Work out the finished part from the listing and answer in its coordinate system (mm). Face numbers are marked on the shaded views. A direction names the side the tool comes from. Coordinates: 2 decimals unless noted, no trailing zeros. Order: outer loops, then holes, each group sorted by start corner. A loop starts at its lowest first (then second) coordinate and runs counter-clockwise, first axis right, second up. Notation, with made-up numbers: (-28.5, 5) -> (-22.5, 5) arc R16 cw to (-22.5, 28) -> close; hole circle Ø11 at (-2, -38.75). An arc over 180 degrees is marked (long way). Use one line per item in the form item = value.
from build123d import *

# Parameters (mm, degrees)
SKETCH1_W                                       = 60
SKETCH1_H                                       = 120
BOSS_EXTRUDE1_DEPTH                             = 6.54
SKETCH10_W                                      = 6.54
SKETCH10_H                                      = 45
BOSS_EXTRUDE5_DEPTH                             = 17
SKETCH17_W                                      = 60
SKETCH17_H                                      = 40
BOSS_EXTRUDE6_DEPTH                             = 29
CUT_EXTRUDE1_REACH                              = 42
CUT_EXTRUDE2_REACH                              = 54.54
SKETCH21_W                                      = 37.9445377
SKETCH21_H                                      = 40
SKETCH23_W                                      = 2
SKETCH23_H                                      = 36
CUT_EXTRUDE3_DEPTH                              = 9
SKETCH24_W                                      = 2
SKETCH24_H                                      = 36
CUT_EXTRUDE4_DEPTH                              = 9
CSK_FOR_M3_FLAT_HEAD_MACHINE_SCREW4_D           = 4.93
CSK_FOR_M3_FLAT_HEAD_MACHINE_SCREW4_DEPTH       = 6.54
CSK_FOR_M3_FLAT_HEAD_MACHINE_SCREW4_CSINK_D     = 12
CSK_FOR_M3_FLAT_HEAD_MACHINE_SCREW4_CSINK_ANGLE = 90
CSK_FOR_M3_FLAT_HEAD_MACHINE_SCREW5_D           = 4.93
CSK_FOR_M3_FLAT_HEAD_MACHINE_SCREW5_DEPTH       = 6.54
CSK_FOR_M3_FLAT_HEAD_MACHINE_SCREW5_CSINK_D     = 12
CSK_FOR_M3_FLAT_HEAD_MACHINE_SCREW5_CSINK_ANGLE = 90
BOSS_EXTRUDE8_DEPTH                             = 29
SKETCH36_W                                      = 60
SKETCH36_H                                      = 1.8
BOSS_EXTRUDE9_DEPTH                             = 6.5
FILLET1_R                                       = 3
FILLET2_R                                       = 2


with BuildPart() as part:
    # Sketch1 → Boss-Extrude1 (new body)
    with BuildSketch(Plane.XY):
        Rectangle(SKETCH1_W, SKETCH1_H)
    extrude(amount=BOSS_EXTRUDE1_DEPTH)

    # Sketch10 → Boss-Extrude5 (add)
    with BuildSketch(Plane(origin=(0, 0, 0), x_dir=(-1, 0, 0), z_dir=(0, 0, -1))):
        with Locations((23.27, -2.5)):
            Rectangle(SKETCH10_W, SKETCH10_H)
        with Locations((-23.27, -2.5)):
            Rectangle(SKETCH10_W, SKETCH10_H)
    extrude(amount=BOSS_EXTRUDE5_DEPTH)

    # Sketch17 → Boss-Extrude6 (add)
    with BuildSketch(Plane.XY.offset(6.54)):
        with Locations((0, -40)):
            Rectangle(SKETCH17_W, SKETCH17_H)
    extrude(amount=BOSS_EXTRUDE6_DEPTH)

    # Sketch18 → Cut-Extrude1 (cut, up to next)
    with BuildSketch(Plane(origin=(0, -20, 0), x_dir=(1, 0, 0), z_dir=(0, 1, 0)), mode=Mode.PRIVATE) as cut_extrude1_sk1:
        with BuildLine():
            Line((5.334966353, -8.526396136), (21.291300905, -12.825812438))
            add(Edge.make_bspline(
                [(5.334966353, -8.526396136), (-17.854714365, -9.780670981), (-12.49786254, -23.648890313), (-7.141010715, -37.517109645), (13.926544327, -30.768916863), (34.994099369, -24.020724082), (21.291300905, -12.825812438)],
                knots=[1.570796327, 1.570796327, 1.570796327, 3.340987112, 3.340987112, 5.111177898, 5.111177898, 6.881368684, 6.881368684, 6.881368684], degree=2, weights=[1, 0.633215673, 1, 0.633215673, 1, 0.633215673, 1]))
        make_face()
    cut_extrude1_tool1 = extrude(cut_extrude1_sk1.sketch, amount=-CUT_EXTRUDE1_REACH, mode=Mode.PRIVATE) & part.part
    add(cut_extrude1_tool1.solids().sort_by_distance((5.792514, -20, 20.554542))[0], mode=Mode.SUBTRACT)

    # Sketch21 → Cut-Extrude2 (cut, up to next)
    with BuildSketch(Plane.XY.offset(35.54), mode=Mode.PRIVATE) as cut_extrude2_sk1:
        with Locations((5.97226885, -40)):
            Rectangle(SKETCH21_W, SKETCH21_H)
    cut_extrude2_tool1 = extrude(cut_extrude2_sk1.sketch, amount=-CUT_EXTRUDE2_REACH, mode=Mode.PRIVATE) & part.part
    add(cut_extrude2_tool1.solids().sort_by_distance((5.972269, -40, 35.54))[0], mode=Mode.SUBTRACT)

    # Sketch23 → Cut-Extrude3 (cut)
    with BuildSketch(Plane(origin=(-13, 0, 0), x_dir=(0, 0, -1), z_dir=(1, 0, 0))):
        with Locations((-33.04, -40)):
            Rectangle(SKETCH23_W, SKETCH23_H)
    extrude(amount=-CUT_EXTRUDE3_DEPTH, mode=Mode.SUBTRACT)

    # Sketch24 → Cut-Extrude4 (cut)
    with BuildSketch(Plane.ZY.offset(-24.9445377)):
        with Locations((33.04, -40)):
            Rectangle(SKETCH24_W, SKETCH24_H)
    extrude(amount=-CUT_EXTRUDE4_DEPTH, mode=Mode.SUBTRACT)

    # CSK for M3 Flat Head Machine Screw4
    with Locations(Plane(origin=(26.54, -12.5, -10), x_dir=(0, 1, 0), z_dir=(1, 0, 0))):
        with Locations((0, 0), (20, 0)):
            CounterSinkHole(CSK_FOR_M3_FLAT_HEAD_MACHINE_SCREW4_D / 2, CSK_FOR_M3_FLAT_HEAD_MACHINE_SCREW4_CSINK_D / 2, depth=CSK_FOR_M3_FLAT_HEAD_MACHINE_SCREW4_DEPTH, counter_sink_angle=CSK_FOR_M3_FLAT_HEAD_MACHINE_SCREW4_CSINK_ANGLE)

    # CSK for M3 Flat Head Machine Screw5
    with Locations(Plane(origin=(-26.54, -12.5, -10), x_dir=(0, -1, 0), z_dir=(-1, 0, 0))):
        with Locations((0, 0), (-20, 0)):
            CounterSinkHole(CSK_FOR_M3_FLAT_HEAD_MACHINE_SCREW5_D / 2, CSK_FOR_M3_FLAT_HEAD_MACHINE_SCREW5_CSINK_D / 2, depth=CSK_FOR_M3_FLAT_HEAD_MACHINE_SCREW5_DEPTH, counter_sink_angle=CSK_FOR_M3_FLAT_HEAD_MACHINE_SCREW5_CSINK_ANGLE)

    # Sketch7 → Boss-Extrude8 (add)
    with BuildSketch(Plane.XY.offset(6.54)):
        with BuildLine():
            Line((-7, 25.533918981), (-18.684094898, 45.817285768))
            ThreePointArc((-18.684094898, 45.817285768), (-20, 46), (-21.294986864, 45.703352481))
            Line((-21.294986864, 45.703352481), (-30, 29.115374119))
            Line((-30, 29.115374119), (-30, 25.533918981))
            Line((-30, 25.533918981), (-7, 25.533918981))
        make_face()
    extrude(amount=BOSS_EXTRUDE8_DEPTH)

    # Sketch36 → Boss-Extrude9 (add)
    with BuildSketch(Plane.XY.offset(6.54)):
        with Locations((0, 54.4)):
            Rectangle(SKETCH36_W, SKETCH36_H)
    extrude(amount=BOSS_EXTRUDE9_DEPTH)

    # Fillet1
    fillet1_edges = [part.edges().sort_by_distance(p)[0] for p in [
        (-7, 25.533918981, 21.04),
    ]]
    fillet(fillet1_edges, radius=FILLET1_R)

    # Fillet2
    fillet2_edges = [part.edges().sort_by_distance(p)[0] for p in [
        (-30, 25.533918981, 21.04),
    ]]
    fillet(fillet2_edges, radius=FILLET2_R)


solid = part.part
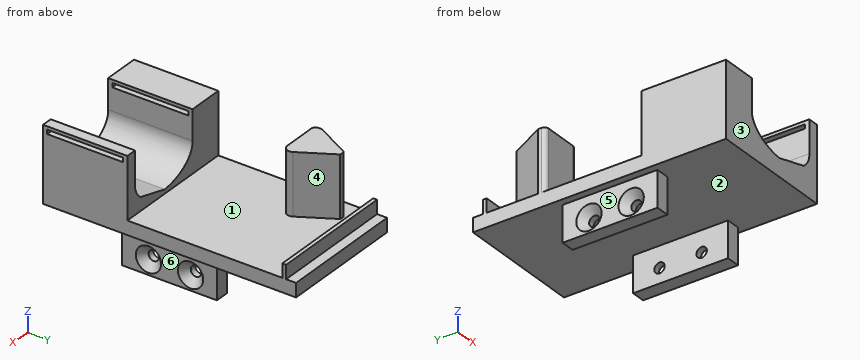
(1) Which of the six approach directions +Z, -Z, +X, -X, +Y, -Y give full straight-line access (tool end or side, diameter ignored) to the marked faces 4, 5 and 6?
Data:
face_4 = +Z, +X
face_5 = -Z, -X, +Y, -Y
face_6 = -Z, +X, +Y, -Y
(2) Section D-D on x = 6.5 is taken. Write down the section's boundary in (y, z), plus the area to 3 significant figures.
Data:
outline = (-60, 0) -> (60, 0) -> (60, 6.54) -> (55.3, 6.54) -> (55.3, 13.04) -> (53.5, 13.04) -> (53.5, 6.54) -> (-20, 6.54) -> (-20, 8.84) -> (-60, 8.84) -> close
area = 889 mm²
(3) Section B-B on z = -10 is taken. Count the separate pieces of the cut face and the enclosed holes in it, plus the area to 3 significant figures.
Data:
separate_pieces = 6
enclosed_holes = 0
area = 410 mm²
(4) Straight lines are drawn through the part: line 1 along Y through (x, z) = (-21.5, -10) (3 decimals); line 2 along Z through (x, y) = (20.95, 7.5) (3 decimals); line 3 along X through (y, z) = (-27.5, 28.5). For each, find the intervals that lie inside material, in ascending order.
Data:
line_1 = -25 to -14.965, -10.035 to 5.035, 9.965 to 20
line_2 = -17 to -12.465, -7.535 to 6.54
line_3 = -30 to -13, 24.94 to 30
(5) The mould has two halves that part along Y. Classify the marked faces 1, 2 and 3: released by +Y, released by -Y, zero draft, split by the parting line, or undercut.
Data:
face_1 = undercut
face_2 = zero draft
face_3 = released by -Y
(6) Each of these flat-tipped pins is pushed along its axis until it touches: P1, Ø2, axis at x = 4.5, y = 37, coming from the -Z side; P2, Ø8.5, axis at x = -9, z = 23.5, coming from the +Y side; P3, Ø5, axis at y = 3.5, z = -9.5, coming from the -X side. Where does it stop, or does it pass through?
Data:
P1 = 0
P2 = 36.38
P3 = -26.54
(7) Section C-C on y = 7.5 is taken. Write down the section's boundary in (x, z) (3 decimals).
Data:
outline = (-30, 0) -> (-26.54, 0) -> (-26.54, -4) -> (-23.005, -7.535) -> (-20, -7.535) -> (-20, 0) -> (20, 0) -> (20, -7.535) -> (23.005, -7.535) -> (26.54, -4) -> (26.54, 0) -> (30, 0) -> (30, 6.54) -> (-30, 6.54) -> close; (-26.54, -17) -> (-20, -17) -> (-20, -12.465) -> (-23.005, -12.465) -> (-26.54, -16) -> close; (20, -17) -> (26.54, -17) -> (26.54, -16) -> (23.005, -12.465) -> (20, -12.465) -> close
(8) Section A-A on z = 24 is taken. Write down the section's boundary in (x, y), plus the area to 3 significant figures.
Data:
outline = (-30, -60) -> (-13, -60) -> (-13, -20) -> (-30, -20) -> close; (-30, 27.53) arc R2 ccw to (-28, 25.53) -> (-12.19, 25.53) arc R3 ccw to (-9.59, 30.03) -> (-18.68, 45.82) arc R3.68 ccw to (-21.29, 45.7) -> (-30, 29.12) -> close; (24.94, -60) -> (30, -60) -> (30, -20) -> (24.94, -20) -> close
area = 1,150 mm²
